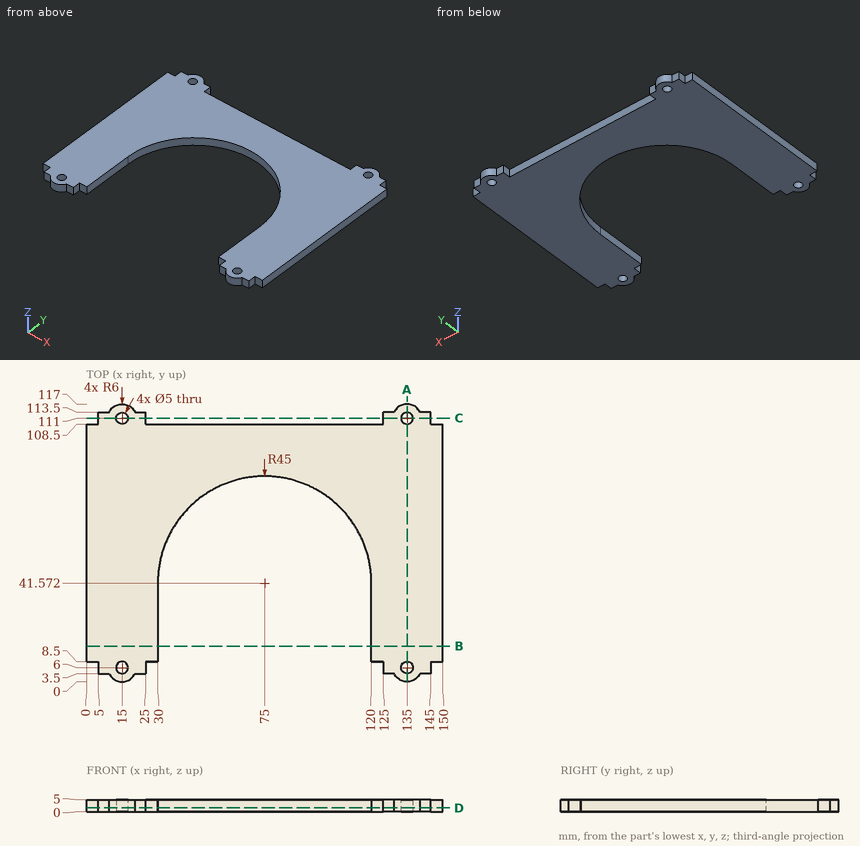
Verification items for this drawing (mm, ordinates from the low corner). Give positions to 0.01 mm unless a question says otherwise; leave off trailing zeros. Loops run counter-clockwise (first coordinate to the right, second up) from the corner with the lowest first, then second, coordinate; pieces in that order, holes last.
1. Cross-section at D-D on z = 1.6. Count the separate pieces of the cut face and the enclosed holes in it, and give its area (3 significant figures).
Derived:
separate pieces: 1
enclosed holes: 4
area: 9,270 mm2
2. Cross-section at B-B on y = 15. Record the cut outline in (x, z).
Derived:
outline: (0, 0) - (30, 0) - (30, 5) - (0, 5) - close; (120, 0) - (150, 0) - (150, 5) - (120, 5) - close
3. Cross-section at C-C on y = 111. Record the cut outline in (x, z), and give its area (3 significant figures).
Derived:
outline: (5, 0) - (12.5, 0) - (12.5, 5) - (5, 5) - close; (17.5, 0) - (25, 0) - (25, 5) - (17.5, 5) - close; (125, 0) - (132.5, 0) - (132.5, 5) - (125, 5) - close; (137.5, 0) - (145, 0) - (145, 5) - (137.5, 5) - close
area: 150 mm2
4. Go/stop test with flat-tipped pins: P1, Ø3, axis at x = 95, z = 3.5, coming from the -Y side; P2, Ø5, axis at x = 39.5, y = 87, coming from the -Z side; P3, Ø4.5, axis at x = 135, y = 111, coming from the -Z side; P4, Ø1, axis at x = 48.5, z = 1, coming from the +Y side. Record where each tip stops, or that it passes through.
Derived:
P1: stops at y = 81.1
P2: stops at z = 0
P3: passes through
P4: stops at y = 108.5
5. Cross-section at A-A on x = 135. Record the cut outline in (y, z).
Derived:
outline: (0, 0) - (3.5, 0) - (3.5, 5) - (0, 5) - close; (8.5, 0) - (108.5, 0) - (108.5, 5) - (8.5, 5) - close; (113.5, 0) - (117, 0) - (117, 5) - (113.5, 5) - close
6. Material ranges on probe 1 along Y at (x, z) = (135, 1.55); probe 2 along X at (y, z) = (111, 3.2); probe 3 along X at (y, z) = (25, 2.6), recorded low to high.
Derived:
probe 1: y = 0 to 3.5, 8.5 to 108.5, 113.5 to 117
probe 2: x = 5 to 12.5, 17.5 to 25, 125 to 132.5, 137.5 to 145
probe 3: x = 0 to 30, 120 to 150
